Can you work these out from the model? Positions are in its coordinate system, mm. A direction names the side the tool comes from. Coordinates: 2 decimals unless noted, no trailing zeros. Loops run counter-clockwise (first coordinate to the right, second up) from the corner with the lowest first, then second, coordinate; pieces in that order, holes last. Notation, with made-up numbers: M 78.5,46.5 L 82.5,46.5 A24 cw 82.5,81.5 Z; hole C 23,-14 d9. An arc over 180 degrees is marked long. Answer as a JSON object with one key per item and string values. Group by question number.
Item 1: We'd pull the mould along Z, two halves only. Please class faces 4 (the cylindrical face through (-37.151, 32.382, 16.843)), 5 (the flat face through (-34.63, -12, 20)), 6 (the cylindrical face through (-37.62, -7.21, 22.89)): +Z half, -Z half, draft (parallel to the pull), parting line (faces both ways), or undercut.
Item 2: I'm going to push flat-ended pins straight in: pin 1 Ø12 at (x, z) = (-7.5, -14.5) entering from +Y; pin 2 Ø5 at (x, z) = (-32, 13) entering from -Y; pin 3 Ø3 at (x, y) = (-33.5, 2.5) entering from +Z; pin 4 Ø22 at (y, z) = (12.5, 11.5) entering from +X. Where does each tip first touch, or does it pass through?
Item 3: Which directions (+Z, -Z, +X, -X, +Y, -Y) give clear straight access to the entire face, cutting with the end or side of a thin tool? Please do faces 1 (the flat face through (-35.63, 16, 22)), 2 (the flat face through (-36.63, 21.2, 7)), 3 (the conical face through (-9.995, 9.135, -2.029)).
Item 4: Suppose I cut it at D-D (x = -27). Write out the boundary of the cut face in (y, z), then the cut area to 3 significant figures.
Item 5: If I drill on line 1 (Y direction, x = -37.25, z = 0); line 2 (Y direction, x = -28.5, z = -4.5); line 3 (Z direction, x = -32, y = 12), over which ranges is the centre line in solid material (lowest first)?
Item 6: Suppose I cut it at A-A (y = 0). Write out the boundary of the cut face in (x, z), then the cut area to 3 significant figures.
Item 7: Suppose I cut it at C-C (x = -21). Write out the boundary of the cut face in (y, z).
```python
from build123d import *


with BuildPart() as part:
    # Esboço2 → revolução (revolve)
    with BuildSketch(Plane.XY, mode=Mode.PRIVATE) as revolu_o_sk:
        with BuildLine():
            Line((-38.630060783, 24), (-36.630060783, 24))
            Line((-36.630060783, 24), (-36.630060783, 22))
            Line((-36.630060783, 22), (-19.529700637, 4.9))
            Line((-19.529700637, 4.9), (-2.089060783, 10))
            Line((-2.089060783, 10), (-2.089060783, 11))
            Line((-2.089060783, 11), (-14.880094771, 8.343395867))
            ThreePointArc((-14.880094771, 8.343395867), (-19.272729764, 8.856141459), (-23.014659232, 11.21328254))
            Line((-23.014659232, 11.21328254), (-34.630060783, 22.828439462))
            Line((-34.630060783, 22.828439462), (-34.630060783, 27))
            Line((-34.630060783, 27), (-35.630060783, 27))
            Line((-35.630060783, 27), (-35.630060783, 36.5))
            Line((-35.630060783, 36.5), (-38.630060783, 36.5))
            Line((-38.630060783, 36.5), (-38.630060783, 24))
        make_face()
    revolve(revolu_o_sk.sketch.rotate(Axis((-109.349560783, 0, 0), (1, 0, 0)), 90), axis=Axis((-109.349560783, 0, 0), (1, 0, 0)))


solid = part.part
```
From the geometry:
{
 "1": {"face 4": "parting line", "face 5": "draft", "face 6": "undercut"},
 "2": {"pin 1": "y = 5.32", "pin 2": "y = -19.03", "pin 3": "z = 26.96", "pin 4": "x = -2.09"},
 "3": {"face 1": "+X", "face 2": "-X", "face 3": "none"},
 "4": {"outline": "C 0,0 d30.4; hole C 0,0 d24.74", "area": "245 mm2"},
 "5": {"line 1": "-36.5 to -24, 24 to 36.5", "line 2": "-16.08 to -13.12, 13.12 to 16.08", "line 3": "-16.25 to -12.56, 12.56 to 16.25"},
 "6": {"outline": "M -38.63,-36.5 L -35.63,-36.5 L -35.63,-27 L -34.63,-27 L -34.63,-22.83 L -23.01,-11.21 A10 cw -14.88,-8.34 L -2.09,-11 L -2.09,-10 L -19.53,-4.9 L -36.63,-22 L -36.63,-24 L -38.63,-24 Z; M -38.63,24 L -36.63,24 L -36.63,22 L -19.53,4.9 L -2.09,10 L -2.09,11 L -14.88,8.34 A10 cw -23.01,11.21 L -34.63,22.83 L -34.63,27 L -35.63,27 L -35.63,36.5 L -38.63,36.5 Z", "area": "248 mm2"},
 "7": {"outline": "C 0,0 d19.32; hole C 0,0 d12.74"}
}
